Input: dimensioned drawing with shaded views. Units: mm. Origin: part minimum x, y, z. A direction names the side the tool comes from. Coordinates: 2 decimals unless noted, no trailing zeros. Order: outer loops, then holes, each group sorted by start corner. A loop starts at its lowest first (then second) coordinate and runs counter-clockwise, first axis right, second up.
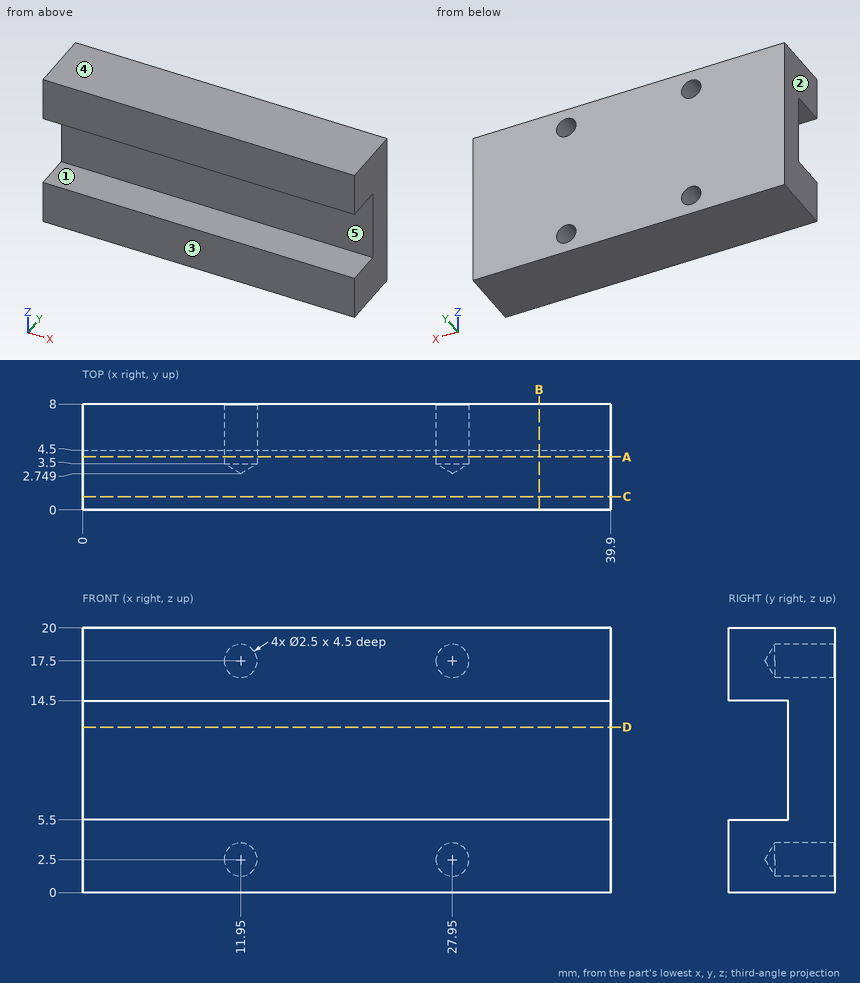
1. Ray query, line 1 (X direction, y = 7, z = 2.5); line 2 (Z direction, x = 11.95, y = 5.45); line 3 (Z direction, x = 3.5, y = 3.5). Return the intervals inside material, ascending.
Findings:
line 1: x = 0 to 10.7, 13.2 to 26.7, 29.2 to 39.9
line 2: z = 0 to 1.25, 3.75 to 16.25, 18.75 to 20
line 3: z = 0 to 5.5, 14.5 to 20
2. Pin query (flat end, axial travel): P1, Ø1.5, axis at x = 11.95, z = 2.5, coming from the +Y side; P2, Ø2, axis at x = 27.95, z = 2.5, coming from the +Y side. Return the tip coordinate at first contact, or that it passes through.
Findings:
P1: stops at y = 3.2
P2: stops at y = 3.35
3. Section query B-B on x = 34.5. Return loops of the section in (y, z), plus the area to 4 significant figures.
Findings:
outline: (0, 0) - (8, 0) - (8, 20) - (0, 20) - (0, 14.5) - (4.5, 14.5) - (4.5, 5.5) - (0, 5.5) - close
area: 119.5 mm2
4. Section query C-C on y = 1. Return loops of the section in (x, z).
Findings:
outline: (0, 0) - (39.9, 0) - (39.9, 5.5) - (0, 5.5) - close; (0, 14.5) - (39.9, 14.5) - (39.9, 20) - (0, 20) - close
5. Section query A-A on y = 4. Return loops of the section in (x, z).
Findings:
outline: (0, 0) - (39.9, 0) - (39.9, 5.5) - (0, 5.5) - close; (0, 14.5) - (39.9, 14.5) - (39.9, 20) - (0, 20) - close; hole circle Ø2.5 at (11.95, 2.5); hole circle Ø2.5 at (11.95, 17.5); hole circle Ø2.5 at (27.95, 2.5); hole circle Ø2.5 at (27.95, 17.5)
6. Section query D-D on z = 12.5. Return loops of the section in (x, y).
Findings:
outline: (0, 4.5) - (39.9, 4.5) - (39.9, 8) - (0, 8) - close
7. Draft query along Z for the marked faces 3, 4 and 5. Return one class per face: released by +Z, released by -Z, zero draft, split by the parting line, or undercut.
Findings:
face 3: zero draft
face 4: released by +Z
face 5: undercut
8. Access query for the marked faces 1 and 2. Directions: +Z, -Z, +X, -X, +Y, -Y. A direction counts if a zero-diameter tool reaches every point of the face in a straight line with its end or side. Return the directions, or none.
Findings:
face 1: +X, -X, -Y
face 2: +Z, -Z, -X, +Y, -Y
